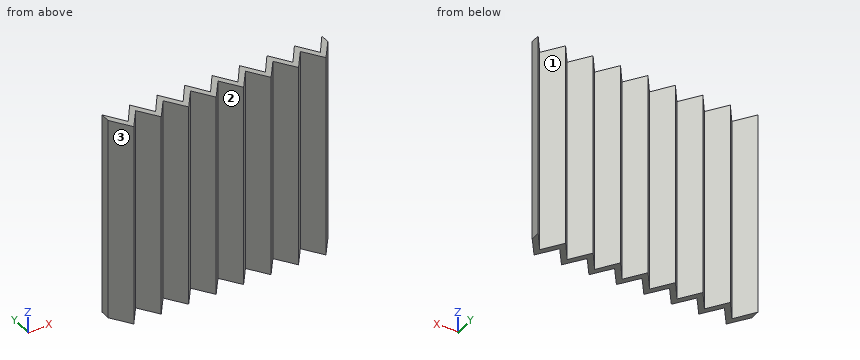
```python
from build123d import *

# Parameters (mm, degrees)
F1_DEPTH = 190.5


with BuildPart() as f1:
    # F0 (on Top) → F1 (new body)
    with BuildSketch(Plane.XY):
        Polygon((-50.8, 0), (-63.5, 18.276649), (-63.5, 9.374281), (-50.8, -8.384577), (-38.1, 9.374281), (-25.4, -8.384577), (-12.7, 9.374281), (0, -8.384577), (12.7, 9.374281), (25.4, -8.384577), (38.1, 9.374281), (50.8, -8.384577), (63.5, 9.374281), (76.2, -8.384577), (88.9, 9.374281), (101.6, -8.384577), (114.3, 9.374281), (127, -8.384577), (139.7, 9.374281), (139.7, 18.276649), (127, 0), (114.3, 18.276649), (101.6, 0), (88.9, 18.276649), (76.2, 0), (63.5, 18.276649), (50.8, 0), (38.1, 18.276649), (25.4, 0), (12.7, 18.276649), (0, 0), (-12.7, 18.276649), (-25.4, 0), (-38.1, 18.276649), align=None)
    extrude(amount=F1_DEPTH)


solid = f1.part
```
The model under review builds one solid part; all positions refer to its coordinate system, in mm. Face numbers are marked on the shaded views. A direction names the side the tool comes from. Coordinates: 2 decimals unless noted, no trailing zeros. Write each loop counter-clockwise with the first axis right and the second up, starting at its lowest first coordinate (ties: lowest second). Pieces come first, ordered by that corner, then holes.
1) Clearance check with flat-ended pins moving along their axes: pin 1 Ø3 at (x, z) = (-27, 128) entering from +Y; pin 2 Ø10 at (x, z) = (-16, 88.5) entering from +Y; pin 3 Ø6 at (y, z) = (-3.5, 105) entering from -X. State where each tip first meets the part, or that it passes through.
2) We need section D-D on x = 95. State the section outline as (y, z) points, then the cut area to 3 significant figures.
3) Machinability: for the marked faces 1, 2 and 3, which of the approach directions +Z, -Z, +X, -X, +Y, -Y give a long, thin tool a straight path to every point of the face, cutting with its end or side? Answer none if there is none.
4) To check wall thickness, follow probe 1 along Y at (x, z) = (-6.5, 49.5); probe 2 along Y at (x, z) = (79, 146). State the ranges of each line that lie inside material, in increasing order.
5) We need section A-A on y = -3.75. Count the separate pieces of the cut face and the enclosed holes in it, then the cut area to 3 significant figures.
Answer list:
1. pin 1: stops at y = 4.46
1. pin 2: stops at y = 18.28
1. pin 3: stops at x = -56.44
2. outline: (0.84, 0) - (9.5, 0) - (9.5, 190.5) - (0.84, 190.5) - close
2. area: 1,650 mm2
3. face 1: +Z, -Z, +Y
3. face 2: +Z, -Z, -Y
3. face 3: +Z, -Z, -X, -Y
4. probe 1: y = 0.7 to 9.35
4. probe 2: y = -4.47 to 4.03
5. separate pieces: 8
5. enclosed holes: 0
5. area: 10,100 mm2
